Solid Edge part; units mm, degrees
sketch "Sketch1" plane through (0, 0, 0) normal (0, 0, 1) x (1, 0, 0)
  circle A0 centre (0, 0) radius 1.5
extrude "Protrusion1" add sketch "Sketch1" along normal blind 30
sketch "Sketch2" plane through (0, 0, 30) normal (0, 0, 1) x (1, 0, 0)
  circle A0 centre (0, 0) radius 3
extrude "ExtrudedProtrusion_2" add sketch "Sketch2" along normal blind 1.75
chamfer "Chamfer_1" distance 1.75 angle 45 1 edges at (-3, 0, 30)
sketch "Sketch3" plane through (0, 0, 31.75) normal (0, 0, 1) x (0, 1, 0)
  line L0 (0.8978, -1.555) -> (1.7956, 0)
  line L1 (1.7956, 0) -> (0.8978, 1.555)
  line L2 (0.8978, 1.555) -> (-0.8978, 1.555)
  line L3 (-0.8978, 1.555) -> (-1.7956, 0)
  line L4 (-1.7956, 0) -> (-0.8978, -1.555)
  line L5 (-0.8978, -1.555) -> (0.8978, -1.555)
extrude "ExtrudedCutout_1" cut sketch "Sketch3" against normal blind 1
sketch "Sketch4" plane through (0, 0, 0) normal (0, 0, -1) x (0, 1, 0)
  circle A0 centre (0, 0) radius 1.6599
extrude "ExtrudedCutout_2" cut sketch "Sketch4" against normal blind 1.75
properties material "Iron, grey cast type 20"
Geometry check sheet. Reference: the model listing, model coordinates, mm. A direction names the side the tool comes from. Round coordinates to 2 decimals unless told otherwise and drop trailing zeros. Order: outer loops, then holes, each group sorted by start corner. A loop starts at its lowest first (then second) coordinate and runs counter-clockwise, first axis right, second up. Notation, with made-up numbers: (-23, 11.25) - (8, 11.25) arc R34 cw to (8, 41.25) - close; hole circle Ø1 at (37, 71). An arc over 180 degrees is marked (long way). Use a Markdown table: item, result. Add a question column.
1) Set-up check for faces 4 (the flat face through (0, 0, 30.75)), 5 (the flat face through (1.3, -1.3, 31.75)): record each of +Z, -Z, +X, -X, +Y, -Y from which the full face is reachable in a straight line by a thin tool's end or side.
2) Section check A-A (y = 0). Record the cut outline in (x, z) (3 decimals), then the cut area to 3 significant figures.
3) Mould release check, pull along Y, two halves, no side actions. Record for faces 1 (the cylindrical face through (-1.5, -0.07, 15.8)), 2 (the flat face through (0, 0, 1.75)), 3 (the flat face through (1.555, 0, 31)): released by +Y, released by -Y, zero draft, split by the parting line, or undercut.
4) Gauge pin test, flat ends, axial feed: P1, Ø2, axis at y = 1, z = 7, coming from the -X side; P2, Ø0.5, axis at y = -0.5, z = 31, coming from the -X side; P3, Ø1.1, axis at y = 0.5, z = 31, coming from the +X side. Record the tip position at first contact, or that the pin passes through.
5) Section check B-B (z = 27). Record the cut outline in (x, y).
6) Thickness scan on line 1 along Z through (x, y) = (0.3, 0.5); line 2 along Y through (x, z) = (-0.25, 4.75); line 3 along Y through (x, z) = (1.25, 10.75). Record the ranges inside material, lowest first.
Established:
| question | item | result |
|---|---|---|
| 1 | face 4 | +Z |
| 1 | face 5 | +Z, +X, -X, +Y, -Y |
| 2 | outline | (-3, 31.75) - (-1.5, 30.25) - (-1.5, 1.75) - (1.5, 1.75) - (1.5, 30.25) - (3, 31.75) - (1.555, 31.75) - (1.555, 30.75) - (-1.555, 30.75) - (-1.555, 31.75) - close |
| 2 | area | 89.1 mm2 |
| 3 | face 1 | split by the parting line |
| 3 | face 2 | zero draft |
| 3 | face 3 | undercut |
| 4 | P1 | x = -1.5 |
| 4 | P2 | x = -2.45 |
| 4 | P3 | x = 2.76 |
| 5 | outline | circle Ø3 at (0, 0) |
| 6 | line 1 | 1.75 to 30.75 |
| 6 | line 2 | -1.48 to 1.48 |
| 6 | line 3 | -0.83 to 0.83 |
